Check sheet for the drawn part. Datum: minimum x, y, z corner. Units: mm. A direction names the side the tool comes from. Give positions to 0.01 mm unless a question says otherwise; leave off trailing zeros. Write each loop counter-clockwise with the first axis right and the second up, starting at its lowest first coordinate (ties: lowest second). Pieces come first, ordered by that corner, then holes. Notation, with made-up numbers: M 1,-19.75 L 30,-19.75 A23 ccw 30,6.25 Z; hole C 80,34.5 d1. An arc over 180 degrees is marked long. Write item = value, one per line. Start each with the question number.
1) Scan lines: L1, parallel to Y at x = 1.8, z = 3.95; L2, parallel to Z at x = 6, y = 11; L3, parallel to X at y = 3, z = 4.5. Record each from-to range of solid material in increasing order.
2) Sectioned sample at C-C, the plane x = 6.5. Record the cut outline in (y, z), then the cut area to 3 significant figures.
3) Set-up check for the marked faces 5, 6 and 7: record each of +Z, -Z, +X, -X, +Y, -Y from which the full face is reachable in a straight line by a thin tool's end or side.
4) Sectioned sample at B-B, the plane y = 7. Record the cut outline in (x, z).
5) Sectioned sample at D-D, the plane y = 16.5. Record the cut outline in (x, z).
6) Gauge pin test, flat ends, axial feed: pin 1 (2.5 mm diameter, centred on x = 2.5, z = 5, fed in from -Y); pin 2 (1.5 mm diameter, centred on y = 2.5, z = 5.5, fed in from +X); pin 3 (1.2 mm diameter, centred on x = 1.8, y = 1.8, fed in from +Z). Record the tip position at first contact, or that the pin passes through.
7) Sectioned sample at A-A, the plane z = 4.75. Record the cut outline in (x, y).
8) Draft check along Y on the marked faces 1, 2, 3 and 4. Enter one of: pulls with the +Y half, pulls with the -Y half, needs draft (parallel to the pull), parting line crosses it, or undercut.
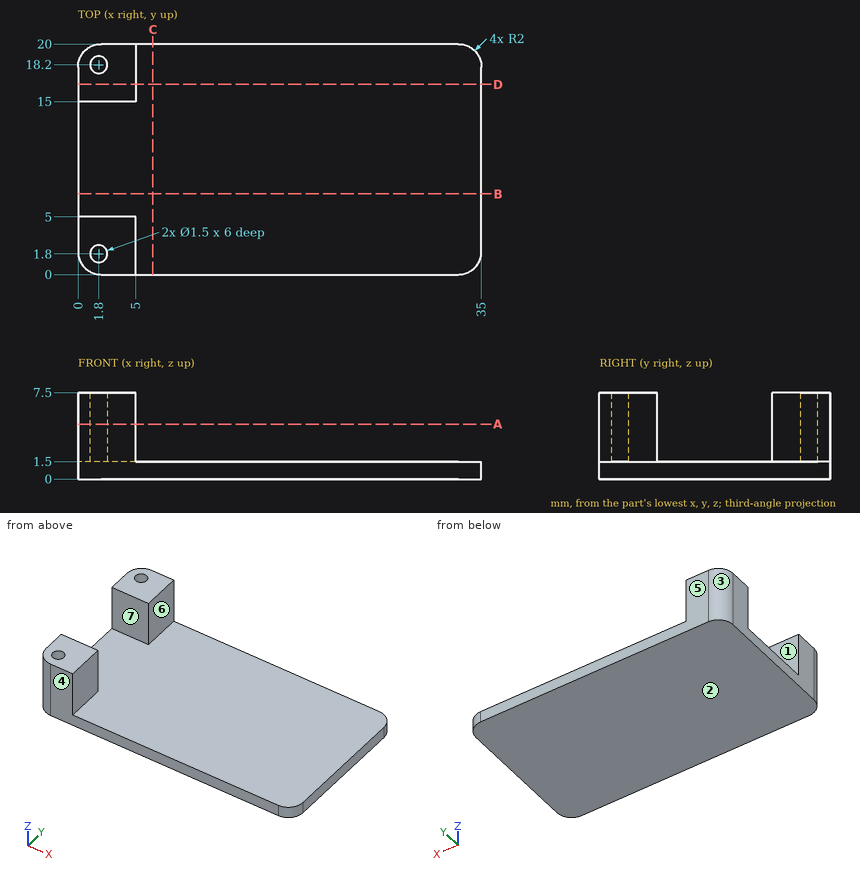
Data:
q1.L1 = 0.01 to 1.05, 2.55 to 5, 15 to 17.45, 18.95 to 19.99
q1.L2 = 0 to 1.5
q1.L3 = 0 to 5
q2.outline = M 0,0 L 20,0 L 20,1.5 L 0,1.5 Z
q2.area = 30.0 mm2
q3.face_5 = +Z, -Z, +X, -X, +Y
q3.face_6 = +Z, +X, +Y, -Y
q3.face_7 = +Z, +X, -X
q4.outline = M 0,0 L 35,0 L 35,1.5 L 0,1.5 Z
q5.outline = M 0,0 L 35,0 L 35,1.5 L 5,1.5 L 5,7.5 L 0,7.5 Z
q6.pin_1 = 0
q6.pin_2 = 5
q6.pin_3 = 1.5
q7.outline = M 0,2 A2 ccw 2,0 L 5,0 L 5,5 L 0,5 Z; M 0,15 L 5,15 L 5,20 L 2,20 A2 ccw 0,18 Z; hole C 1.8,1.8 d1.5; hole C 1.8,18.2 d1.5
q8.face_1 = undercut
q8.face_2 = needs draft
q8.face_3 = pulls with the +Y half
q8.face_4 = pulls with the -Y half
